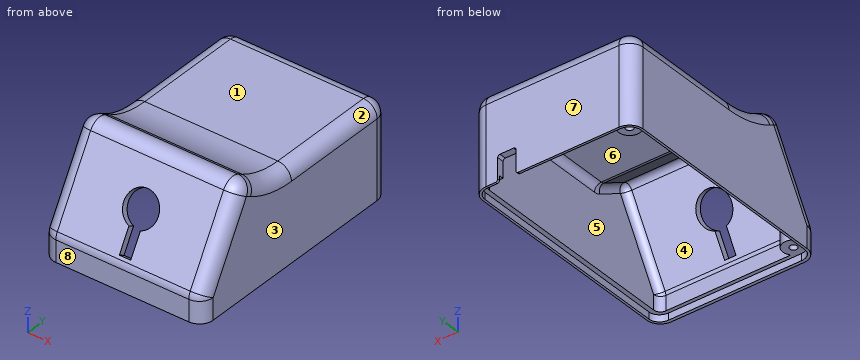
```python
from build123d import *

# Parameters (mm, degrees)
SKETCH1_W           = 32.2
SKETCH1_H           = 21
BOSS_EXTRUDE2_DEPTH = 1.5
BOSS_EXTRUDE3_DEPTH = 1.5
BOSS_EXTRUDE4_DEPTH = 1.5
BOSS_EXTRUDE5_DEPTH = 35.2
SKETCH5_W           = 35.2
SKETCH5_H           = 5.556871517
BOSS_EXTRUDE6_DEPTH = 1.5
SKETCH6_W           = 35.2
SKETCH6_H           = 20.226133569
BOSS_EXTRUDE7_DEPTH = 1.5
FILLET3_R           = 20
FILLET_EXTERIOR_R   = 3
FILLET_INTERIOR_R   = 1.5
SKETCH7_W           = 4
SKETCH7_H           = 8.5
CUT_EXTRUDE1_DEPTH  = 1.5
FILLET4_R           = 0.5
CUT_EXTRUDE2_DEPTH  = 1.5
SCREW_BOSS1_REACH   = 41.636
SKETCH10_R          = 2.3
SKETCH10_R_2        = 0.8
SCREW_BOSS2_REACH   = 41.636
SKETCH11_R          = 2.3
SKETCH11_R_2        = 0.8


with BuildPart() as part:
    # Sketch1 → Boss-Extrude2 (new body)
    with BuildSketch(Plane(origin=(0, -25.251844214, 14.579159054), x_dir=(1, 0, 0), z_dir=(3.491481338843128e-15, -0.866025403784445, 0.4999999999999889))):
        with Locations((1.234580757, 10.21530973)):
            Rectangle(SKETCH1_W, SKETCH1_H)
        with BuildLine():
            Line((-0.015419243, 1.21530973), (2.484580757, 1.21530973))
            Line((2.484580757, 1.21530973), (2.484580757, 6.626786357))
            ThreePointArc((2.484580757, 6.626786357), (1.234580757, 14.01530973), (-0.015419243, 6.626786357))
            Line((-0.015419243, 6.626786357), (-0.015419243, 1.21530973))
        make_face(mode=Mode.SUBTRACT)
    extrude(amount=BOSS_EXTRUDE2_DEPTH)

    # Sketch2 → Boss-Extrude3 (add)
    with BuildSketch(Plane(origin=(17.334580757, 0, 0), x_dir=(0, 0, -1), z_dir=(1, 0, 0))):
        Polygon((-15.082610048, -26.693227454), (-9.525738531, -26.693227454), (-9.525738531, 25.295602697), (-28.2518721, 25.295602697), (-28.2518721, -7.503058425), (-33.269143528, -16.193227454), align=None)
    extrude(amount=BOSS_EXTRUDE3_DEPTH)

    # Sketch3 → Boss-Extrude4 (add)
    with BuildSketch(Plane.ZY.offset(14.865419243)):
        Polygon((28.2518721, 25.295602697), (28.2518721, -7.503058425), (33.269143528, -16.193227454), (15.082610048, -26.693227454), (9.525738531, -26.693227454), (9.525738531, 25.295602697), align=None)
    extrude(amount=BOSS_EXTRUDE4_DEPTH)

    # Sketch4 → Boss-Extrude5 (add)
    with BuildSketch(Plane(origin=(18.834580757, 0, 0), x_dir=(0, 0, -1), z_dir=(1, 0, 0))):
        Polygon((-28.2518721, -7.503058425), (-33.269143528, -16.193227454), (-34.568181634, -15.443227454), (-29.7518721, -7.101134637), (-29.7518721, 25.295602697), (-28.2518721, 25.295602697), align=None)
    extrude(amount=-BOSS_EXTRUDE5_DEPTH)

    # Sketch5 → Boss-Extrude6 (add)
    with BuildSketch(Plane.XZ.offset(26.693227454)):
        with Locations((1.234580757, 12.30417429)):
            Rectangle(SKETCH5_W, SKETCH5_H)
    extrude(amount=-BOSS_EXTRUDE6_DEPTH)

    # Sketch6 → Boss-Extrude7 (add)
    with BuildSketch(Plane(origin=(0, 25.295602697, 0), x_dir=(1, 0, 0), z_dir=(0, 1, 0))):
        with Locations((1.234580757, -19.638805316)):
            Rectangle(SKETCH6_W, SKETCH6_H)
    extrude(amount=-BOSS_EXTRUDE7_DEPTH)

    # Fillet3
    fillet3_edges = [part.edges().sort_by_distance(p)[0] for p in [
        (1.234580757, -7.101134637, 29.7518721),
    ]]
    fillet(fillet3_edges, radius=FILLET3_R)

    # Fillet-Exterior
    fillet_exterior_edges = [part.edges().sort_by_distance(p)[0] for p in [
        (-16.365419243, 11.776725954, 29.7518721),
        (18.834580757, -13.592689121, 33.499772829),
        (18.834580757, -6.91853169, 30.433355574),
        (-16.365419243, -6.91853169, 30.433355574),
        (1.234580757, -26.693227454, 15.082610048),
        (18.834580757, -21.068227454, 24.825395841),
        (18.834580757, -26.693227454, 12.30417429),
        (18.834580757, 25.295602697, 19.638805315),
        (-16.365419243, 25.295602697, 19.638805315),
        (-16.365419243, -26.693227454, 12.30417429),
        (-16.365419243, -21.068227454, 24.825395841),
        (1.234580757, -15.443227454, 34.568181634),
        (1.234580757, 25.295602697, 29.7518721),
        (18.834580757, 11.776725954, 29.7518721),
        (-16.365419243, -13.592689121, 33.499772829),
    ]]
    fillet(fillet_exterior_edges, radius=FILLET_EXTERIOR_R)

    # Fillet-Interior
    fillet_interior_edges = [part.edges().sort_by_distance(p)[0] for p in [
        (17.334580757, 8.146272136, 28.2518721),
        (17.334580757, 23.795602697, 18.888805315),
        (-14.865419243, 23.795602697, 18.888805315),
        (1.234580757, 23.795602697, 28.2518721),
        (17.334580757, -11.198623887, 30.385507814),
        (-14.865419243, -11.198623887, 30.385507814),
        (-14.865419243, 8.146272136, 28.2518721),
        (-14.865419243, -20.043708401, 23.599914894),
        (1.234580757, -14.894189349, 32.519143528),
        (1.234580757, -7.503058425, 28.2518721),
        (-14.865419243, -25.193227454, 12.103212395),
        (17.334580757, -20.043708401, 23.599914894),
        (1.234580757, -25.193227454, 14.68068626),
        (17.334580757, -25.193227454, 12.103212395),
    ]]
    fillet(fillet_interior_edges, radius=FILLET_INTERIOR_R)

    # Sketch7 → Cut-Extrude1 (cut)
    with BuildSketch(Plane(origin=(0, 25.295602697, 0), x_dir=(1, 0, 0), z_dir=(0, 1, 0))):
        with Locations((11.239580757, -10.8)):
            Rectangle(SKETCH7_W, SKETCH7_H)
    extrude(amount=-CUT_EXTRUDE1_DEPTH, mode=Mode.SUBTRACT)

    # Fillet4
    fillet4_edges = [part.edges().sort_by_distance(p)[0] for p in [
        (9.239580757, 24.545602697, 9.525738531),
        (9.239580757, 24.545602697, 15.05),
        (13.239580757, 24.545602697, 9.525738531),
        (13.239580757, 24.545602697, 15.05),
    ]]
    fillet(fillet4_edges, radius=FILLET4_R)

    # Sketch9 → Cut-Extrude2 (cut)
    with BuildSketch(Plane(origin=(0, 0, 9.525738531), x_dir=(-1, 0, 0), z_dir=(0, 0, -1))):
        with BuildLine():
            Line((13.365419243, -25.99226556), (-15.834580757, -25.99226556))
            add(Edge.make_bspline(
                [(-15.834580757, -25.99226556), (-16.142981162, -25.99226556), (-16.764416225, -25.886824157), (-17.587620167, -25.41563579), (-18.184470703, -24.656923007), (-18.334580757, -24.010728961), (-18.334580757, -23.693227454)],
                knots=[0, 0, 0, 0, 0.392699082, 0.785398163, 1.178097245, 1.570796327, 1.570796327, 1.570796327, 1.570796327], degree=3))
            Line((-18.334580757, -23.693227454), (-18.334580757, 22.295602697))
            ThreePointArc((-18.334580757, 22.295602697), (-17.60234771, 24.06336965), (-15.834580757, 24.795602697))
            Line((-15.834580757, 24.795602697), (13.365419243, 24.795602697))
            ThreePointArc((13.365419243, 24.795602697), (15.133186196, 24.06336965), (15.865419243, 22.295602697))
            Line((15.865419243, 22.295602697), (15.865419243, -23.693227454))
            add(Edge.make_bspline(
                [(15.865419243, -23.693227454), (15.865419243, -24.010728961), (15.715309189, -24.656923007), (15.118458653, -25.41563579), (14.295254711, -25.886824157), (13.673819649, -25.99226556), (13.365419243, -25.99226556)],
                knots=[1.570796327, 1.570796327, 1.570796327, 1.570796327, 1.963495408, 2.35619449, 2.748893572, 3.141592654, 3.141592654, 3.141592654, 3.141592654], degree=3))
        make_face()
        with BuildLine():
            Line((14.865419243, 22.295602697), (14.865419243, -23.693227454))
            add(Edge.make_bspline(
                [(13.365419243, -24.99226556), (14.865419243, -24.99226556), (14.865419243, -23.693227454)],
                knots=[1.570796327, 1.570796327, 1.570796327, 3.141592654, 3.141592654, 3.141592654], degree=2, weights=[1, 0.707106781, 1]))
            Line((13.365419243, -24.99226556), (-15.834580757, -24.99226556))
            add(Edge.make_bspline(
                [(-17.334580757, -23.693227454), (-17.334580757, -24.99226556), (-15.834580757, -24.99226556)],
                knots=[0, 0, 0, 1.570796327, 1.570796327, 1.570796327], degree=2, weights=[1, 0.707106781, 1]))
            Line((-17.334580757, -23.693227454), (-17.334580757, 22.295602697))
            ThreePointArc((-17.334580757, 22.295602697), (-16.895240929, 23.356262868), (-15.834580757, 23.795602697))
            Line((-15.834580757, 23.795602697), (13.365419243, 23.795602697))
            ThreePointArc((13.365419243, 23.795602697), (14.426079415, 23.356262868), (14.865419243, 22.295602697))
        make_face(mode=Mode.SUBTRACT)
    extrude(amount=-CUT_EXTRUDE2_DEPTH, mode=Mode.SUBTRACT)

    # Screw-Boss1: up to this face of the body (flat: up to its plane)
    screw_boss1_end = Plane(part.part.faces().sort_by_distance((1.234580757, 7.59723403, 28.2518721))[0])
    # Sketch10 → Screw-Boss1 (add, up to the picked face)
    with BuildSketch(Plane(origin=(0, 0, 11.025738531), x_dir=(-1, 0, 0), z_dir=(0, 0, -1)), mode=Mode.PRIVATE) as screw_boss1_sk1:
        with Locations((13.365419243, 22.295602697)):
            Circle(SKETCH10_R)
        with Locations((13.365419243, 22.295602697)):
            Circle(SKETCH10_R_2, mode=Mode.SUBTRACT)
    screw_boss1_tool1 = split(extrude(screw_boss1_sk1.sketch, amount=-SCREW_BOSS1_REACH, mode=Mode.PRIVATE), bisect_by=screw_boss1_end, keep=Keep.BOTH, mode=Mode.PRIVATE)
    add(screw_boss1_tool1.solids().sort_by(Axis((-11.130473, 22.295603, 11.025739), (0, 0, 1)))[0])

    # Screw-Boss2: up to this plane
    screw_boss2_end = Plane(origin=(0, -25.251844214, 14.579159054), z_dir=(3.5680069050429865e-15, -0.8660254037844453, 0.49999999999998884))
    # Sketch11 → Screw-Boss2 (add, up to the surface)
    with BuildSketch(Plane(origin=(0, 0, 11.025738531), x_dir=(-1, 0, 0), z_dir=(0, 0, -1)), mode=Mode.PRIVATE) as screw_boss2_sk1:
        with Locations((13.365419243, -23.693227454)):
            Circle(SKETCH11_R)
        with Locations((13.365419243, -23.693227454)):
            Circle(SKETCH11_R_2, mode=Mode.SUBTRACT)
    screw_boss2_tool1 = split(extrude(screw_boss2_sk1.sketch, amount=-SCREW_BOSS2_REACH, mode=Mode.PRIVATE), bisect_by=screw_boss2_end, keep=Keep.BOTH, mode=Mode.PRIVATE)
    add(screw_boss2_tool1.solids().sort_by_distance((-11.130473, -23.693227, 11.025739))[0])


solid = part.part
```
Check sheet for the modelled part. Datum: model origin and axes. Units: mm. Face numbers are marked on the shaded views. A direction names the side the tool comes from. Round coordinates to 2 decimals unless told otherwise and drop trailing zeros. Loops run counter-clockwise (first coordinate to the right, second up) from the corner with the lowest first, then second, coordinate; pieces in that order, holes last. Notation, with made-up numbers: (-25, -37.5) - (15, -37.5) arc R15 ccw to (15, -13.5) - close; hole circle Ø2 at (73, 24). An arc over 180 degrees is marked (long way). Write item = value, one per line. Start each with the question number.
Q1. Access from +Z, -Z, +X, -X, +Y, -Y to the whole of each face (thin tool, end or side, straight path). Record for the marked faces 1, 2, 3 and 4.
Q2. Depth check by flat-ended pin: P1, Ø3, axis at y = -23.5, z = 18, coming from the -X side; P2, Ø12.5, axis at x = 1.5, z = 18.5, coming from the -Y side; P3, Ø3, axis at y = -24, z = 19, coming from the +X side; P4, Ø1, axis at x = 7, y = -17, coming from the -Z side. Enter the tip coordinate at first touch or a pass-through.
Q3. Section check A-A (y = 9). Record the boundary of the cut face in (x, z).
Q4. Thickness scan on L1, parallel to X at y = -10.5, z = 14; L2, parallel to X at y = -9, z = 10.5; L3, parallel to Y at x = -11.5, z = 20. Record the ranges inside material, lowest first.
Q5. Release check for a two-part mould opening along Y. For the marked faces 5, 6, 7 and 8 record: pulls with the +Y half, pulls with the -Y half, needs draft (parallel to the pull), parting line crosses it, or undercut.
Derived:
q1.face_1 = +Z, +X, -X, +Y
q1.face_2 = +Z, +X, +Y
q1.face_3 = +Z, -Z, +X, +Y, -Y
q1.face_4 = -Z
q2.P1 = -16.36
q2.P2 = -26.69
q2.P3 = 18.62
q2.P4 = 28.01
q3.outline = (-16.37, 9.53) - (-15.87, 9.53) - (-15.87, 11.03) - (-14.87, 11.03) - (-14.87, 26.75) arc R1.5 cw to (-13.37, 28.25) - (15.83, 28.25) arc R1.5 cw to (17.33, 26.75) - (17.33, 11.03) - (18.33, 11.03) - (18.33, 9.53) - (18.83, 9.53) - (18.83, 26.75) arc R3 ccw to (15.83, 29.75) - (-13.37, 29.75) arc R3 ccw to (-16.37, 26.75) - close
q4.L1 = -16.37 to -14.87, 17.33 to 18.83
q4.L2 = -16.37 to -15.87, 18.33 to 18.83
q4.L3 = -23.85 to -22.12, 20.95 to 23.64, 23.8 to 25.3
q5.face_5 = undercut
q5.face_6 = undercut
q5.face_7 = pulls with the +Y half
q5.face_8 = pulls with the -Y half
